Here's the drawing with two shaded views (mm, measured from the low corner). I have some questions. A direction names the side the tool comes from. Give positions to 0.01 mm unless a question says otherwise; leave off trailing zeros. Write each loop counter-clockwise with the first axis right and the second up, starting at its lowest first coordinate (ties: lowest second). Pieces come first, ordered by that corner, then holes. Notation, with made-up numbers: (78.5, 52.25) - (110.5, 52.25) arc R33 ccw to (110.5, 80.25) - close; hole circle Ø2 at (32.5, -35.75). An arc over 180 degrees is marked (long way). Answer as a JSON object with one key per item and string values. Group by question number.
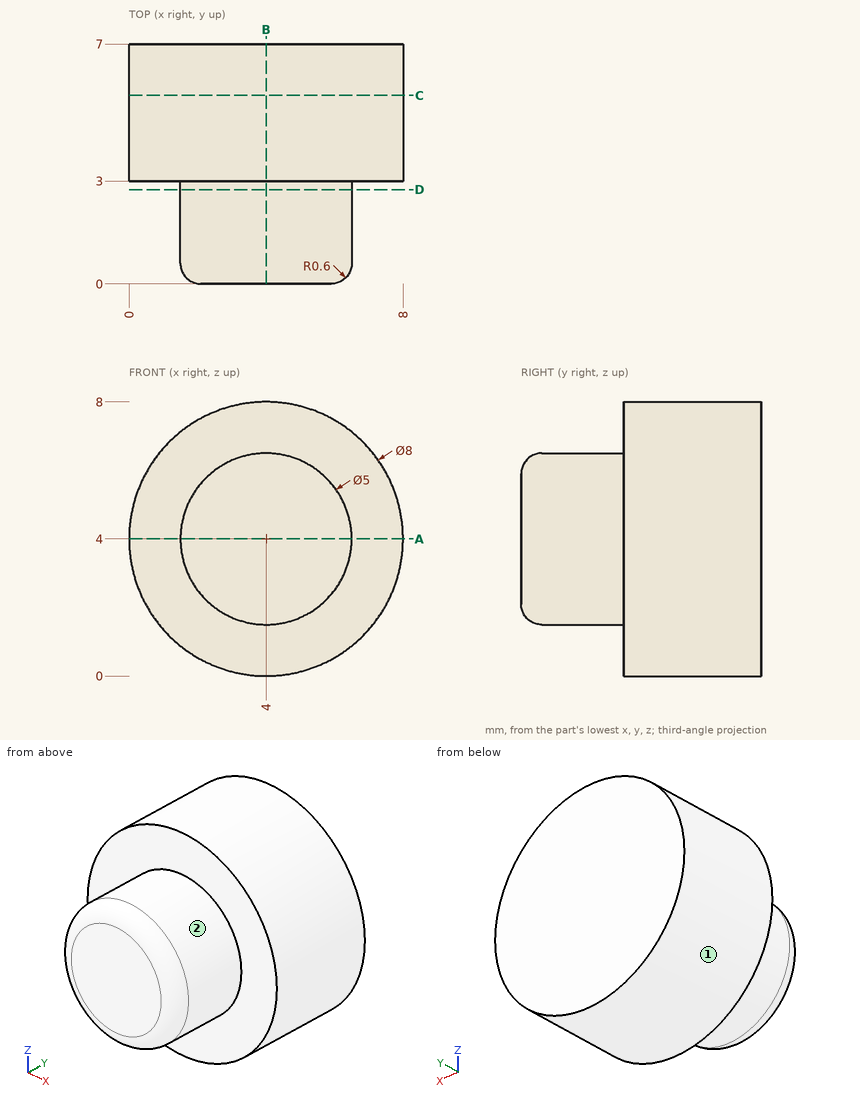
(1) I need wall thicknesses on L1, parallel to Y at x = 5.5, z = 6.75; L2, parallel to Y at x = 2.5, z = 2.75; L3, parallel to X at y = 5.25, z = 5.5. Which ranges of each line are inside material? Lowest first, please.
(2) I want a section at A-A, the plane z = 4. Please give me the cut outline in (x, y), and give its area (3 significant figures).
(3) I want a section at D-D, the plane y = 2.75. Please give me the cut outline in (x, z).
(4) Will this pin go through, and if not, where does the flat tip stop? P1, Ø2, axis at x = 6.5, y = 3.5, coming from the -Z side.
(5) I want a section at B-B, the plane x = 4. Please give me the cut outline in (y, z).
(6) I want a section at C-C, the plane y = 5.5. Please give me the cut outline in (x, z), and give its area (3 significant figures).
(7) For the marked faces 1 and 2, which set-ups out of +Z, -Z, +X, -X, +Y, -Y let a thin tool reach every point of the face, with its end or its side?
Entries:
{
 "1": {"L1": "3 to 7", "L2": "0 to 7", "L3": "0.29 to 7.71"},
 "2": {"outline": "(0, 3) - (1.5, 3) - (1.5, 0.6) arc R0.6 ccw to (2.1, 0) - (5.9, 0) arc R0.6 ccw to (6.5, 0.6) - (6.5, 3) - (8, 3) - (8, 7) - (0, 7) - close", "area": "46.8 mm^2"},
 "3": {"outline": "circle Ø5 at (4, 4)"},
 "4": {"P1": "z = 0.29"},
 "5": {"outline": "(0, 2.1) arc R0.6 ccw to (0.6, 1.5) - (3, 1.5) - (3, 0) - (7, 0) - (7, 8) - (3, 8) - (3, 6.5) - (0.6, 6.5) arc R0.6 ccw to (0, 5.9) - close"},
 "6": {"outline": "circle Ø8 at (4, 4)", "area": "50.3 mm^2"},
 "7": {"face 1": "+Y, -Y", "face 2": "-Y"}
}
